For this review, take the finished solid that the model builds, in its own axes (mm). Face numbers are marked on the shaded views. A direction names the side the tool comes from. Coordinates: 2 decimals unless noted, no trailing zeros. Loops run counter-clockwise (first coordinate to the right, second up) from the corner with the lowest first, then second, coordinate; pieces in that order, holes last. Notation, with made-up numbers: (-36, 45.5) -> (-24, 45.5) arc R35 cw to (-24, 84.5) -> close; hole circle Ø4 at (-21.75, 43.25). An arc over 180 degrees is marked (long way). One line per item, written item: value.
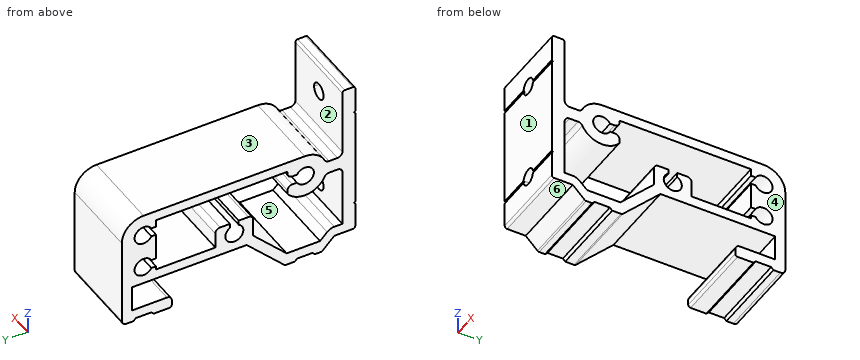
from build123d import *

# Parameters (mm, degrees)
F1_DEPTH = 25.4
F3_DEPTH = 25.4


# Not quite as in the source:
# - ends of sketch curves that miss each other by under 0.0002 mm in the source are joined


with BuildPart() as f1:
    # F0 (on Right) → F1 (new body)
    with BuildSketch(Plane.YZ):
        with BuildLine():
            Line((-36.7665, 26.0985), (-36.7665, 18.2245))
            Line((-36.7665, 18.2245), (-36.3855, 17.8435))
            Line((-36.3855, 17.8435), (-36.7665, 17.4625))
            Line((-36.7665, 17.4625), (-36.7665, -13.5255))
            Line((-36.7665, -13.5255), (-36.3855, -13.9065))
            Line((-36.3855, -13.9065), (-36.7665, -14.2875))
            Line((-36.7665, -14.2875), (-36.7665, -22.1615))
            ThreePointArc((-36.7665, -22.1615), (-36.5433153673, -22.7003153673), (-36.0045, -22.9235))
            Line((-36.0045, -22.9235), (-30.1625, -22.9235))
            Line((-30.1625, -22.9235), (-26.4486898, -26.6373356))
            ThreePointArc((-26.4486898, -26.6373356), (-26.2014589755, -26.8024962038), (-25.9098542, -26.8605))
            Line((-25.9098542, -26.8605), (-24.0665, -26.8605))
            Line((-24.0665, -26.8605), (-23.3045, -26.0985))
            Line((-23.3045, -26.0985), (-18.4785, -26.0985))
            Line((-18.4785, -26.0985), (-17.7165, -26.8605))
            Line((-17.7165, -26.8605), (-14.9389846, -26.8605))
            ThreePointArc((-14.9389846, -26.8605), (-14.6473881211, -26.8024996403), (-14.4001819327, -26.6373280669))
            Line((-14.4001819327, -26.6373280669), (-2.5583642, -14.7955))
            Line((-2.5583642, -14.7955), (33.5915, -14.7955))
            Line((33.5915, -14.7955), (33.5915, -22.9235))
            Line((33.5915, -22.9235), (22.5425, -22.9235))
            ThreePointArc((22.5425, -22.9235), (21.4648692655, -23.3698692655), (21.0185, -24.4475))
            Line((21.0185, -24.4475), (21.0185, -26.0985))
            ThreePointArc((21.0185, -26.0985), (21.2416846327, -26.6373153673), (21.7805, -26.8605))
            Line((21.7805, -26.8605), (26.7335, -26.8605))
            Line((26.7335, -26.8605), (27.4955, -26.0985))
            Line((27.4955, -26.0985), (32.3215, -26.0985))
            Line((32.3215, -26.0985), (33.0835, -26.8605))
            Line((33.0835, -26.8605), (35.2425, -26.8605))
            ThreePointArc((35.2425, -26.8605), (36.3201307345, -26.4141307345), (36.7665, -25.3365))
            Line((36.7665, -25.3365), (36.7665, 1.9685))
            ThreePointArc((36.7665, 1.9685), (34.7578383054, 6.8178383054), (29.9085, 8.8265))
            Line((29.9085, 8.8265), (-20.8915, 8.8265))
            ThreePointArc((-20.8915, 8.8265), (-24.5711182212, 7.7557768852), (-27.1017564824, 4.8779464117))
            ThreePointArc((-27.1017564824, 4.8779464117), (-27.6641193484, 4.2384353631), (-28.4818074, 4.0005))
            Line((-28.4818074, 4.0005), (-31.1785, 4.0005))
            ThreePointArc((-31.1785, 4.0005), (-32.2561307345, 4.4468692655), (-32.7025, 5.5245))
            Line((-32.7025, 5.5245), (-32.7025, 26.0985))
            ThreePointArc((-32.7025, 26.0985), (-32.9256846327, 26.6373153673), (-33.4645, 26.8605))
            Line((-33.4645, 26.8605), (-36.0045, 26.8605))
            ThreePointArc((-36.0045, 26.8605), (-36.5433153673, 26.6373153673), (-36.7665, 26.0985))
        make_face()
        with BuildLine():
            Line((-18.4133236, 3.3655), (-16.9545, 3.3655))
            ThreePointArc((-16.9545, 3.3655), (-15.8768692655, 3.8118692655), (-15.4305, 4.8895))
            Line((-15.4305, 4.8895), (-15.4305, 5.6515))
            Line((-15.4305, 5.6515), (25.9715, 5.6515))
            Line((25.9715, 5.6515), (25.9715, 3.3655))
            Line((25.9715, 3.3655), (27.430349, 3.3655))
            ThreePointArc((27.430349, 3.3655), (32.7533, 1.9685), (27.4303420089, 0.5714960589))
            Line((27.4303420089, 0.5714960589), (25.9715, 0.5715))
            Line((25.9715, 0.5715), (25.9715, -7.747))
            Line((25.9715, -7.747), (27.430349, -7.747))
            ThreePointArc((27.430349, -7.747), (32.7533, -9.144), (27.4303420089, -10.5410039411))
            Line((27.4303420089, -10.5410039411), (25.9715, -10.541))
            Line((25.9715, -10.541), (25.9715, -11.6205))
            Line((25.9715, -11.6205), (7.3025, -11.6205))
            Line((7.3025, -11.6205), (7.3025, -6.731))
            ThreePointArc((7.3025, -6.731), (6.8561307345, -5.6533692655), (5.7785, -5.207))
            Line((5.7785, -5.207), (2.7305, -5.207))
            Line((2.7305, -5.207), (2.7305, -6.665849))
            ThreePointArc((2.7305, -6.665849), (1.3335, -11.9888), (-0.0635039411, -6.6658420089))
            Line((-0.0635039411, -6.6658420089), (-0.0635, -5.207))
            Line((-0.0635, -5.207), (-3.1115, -5.207))
            ThreePointArc((-3.1115, -5.207), (-4.1891307345, -5.6533692655), (-4.6355, -6.731))
            Line((-4.6355, -6.731), (-4.6355, -12.3825))
            Line((-4.6355, -12.3825), (-15.1765, -22.9235))
            Line((-15.1765, -22.9235), (-25.6723642, -22.9235))
            Line((-25.6723642, -22.9235), (-27.9174194, -20.6784448))
            ThreePointArc((-27.9174194, -20.6784448), (-28.9474718056, -19.9901859209), (-30.1625, -19.7485))
            Line((-30.1625, -19.7485), (-32.7025, -19.7485))
            Line((-32.7025, -19.7485), (-32.7025, -1.5875))
            ThreePointArc((-32.7025, -1.5875), (-32.2561307345, -0.5098692655), (-31.1785, -0.0635))
            Line((-31.1785, -0.0635), (-28.4818074, -0.0635))
            ThreePointArc((-28.4818074, -0.0635), (-27.6641096434, -0.3014415336), (-27.1017455591, -0.9409666943))
            ThreePointArc((-27.1017455591, -0.9409666943), (-21.615457962, -4.8511809947), (-15.4305020835, -2.1799534173))
            Line((-15.4305020835, -2.1799534173), (-15.4305, -0.9525))
            ThreePointArc((-15.4305, -0.9525), (-15.8768692655, 0.1251307345), (-16.9545, 0.5715))
            Line((-16.9545, 0.5715), (-18.4133236, 0.5715))
            ThreePointArc((-18.4133236, 0.5715), (-23.7363, 1.9685), (-18.4133236, 3.3655))
        make_face(mode=Mode.SUBTRACT)
    extrude(amount=F1_DEPTH)

    # F2 (on face) → F3 (cut)
    with BuildSketch(Plane.XZ.offset(36.7665)):
        with BuildLine():
            ThreePointArc((10.1889011104, 17.4625), (12.8915839509, 15.311811972), (15.24, 17.8445763886))
            ThreePointArc((15.24, 17.8445763886), (12.5084160491, 20.3773408052), (10.1889011104, 17.4625))
        make_face()
        with BuildLine():
            ThreePointArc((10.1887375685, -13.5255), (12.5089588736, -16.4393054185), (15.24, -13.9065))
            ThreePointArc((15.24, -13.9065), (12.8910411264, -11.3736945815), (10.1887375685, -13.5255))
        make_face()
    extrude(amount=-F3_DEPTH, mode=Mode.SUBTRACT)


solid = f1.part
1. Take a section at B-B, the plane z = 16.5. Give the boundary of the cut face in (x, y).
Return value:
outline: (0, -36.77) -> (10.55, -36.77) -> (10.55, -32.7) -> (0, -32.7) -> close; (14.85, -36.77) -> (25.4, -36.77) -> (25.4, -32.7) -> (14.85, -32.7) -> close
2. Insertion check: pin 1 Ø3 at (x, y) = (5, 6) entering from +Z; pin 2 Ø0.8 at (x, z) = (11, -25.5) entering from -Y; pin 3 Ø5 at (x, y) = (12.5, 18) entering from -Z. Each pin has a flat end and moves straight along its axis. Give the tip position at first contact, or say it passes through.
Return value:
pin 1: stops at z = 8.83
pin 2: stops at y = -27.99
pin 3: stops at z = -14.8
3. Take a section at A-A, the plane z = -9. Give the boundary of the cut face in (x, y).
Return value:
outline: (0, -36.77) -> (25.4, -36.77) -> (25.4, -32.7) -> (0, -32.7) -> close; (0, -4.64) -> (25.4, -4.64) -> (25.4, -1.51) -> (0, -1.51) -> close; (0, 4.17) -> (25.4, 4.17) -> (25.4, 7.3) -> (0, 7.3) -> close; (0, 32.75) -> (25.4, 32.75) -> (25.4, 36.77) -> (0, 36.77) -> close
4. For the marked faces 4, 5 and 6, list the 3-axis set-ups (+Z, -Z, +X, -X, +Y, -Y) from which the entire face can be reached by the end or side of a thin tool; tool diameter is ignored.
Return value:
face 4: +Z, -Z, +X, +Y, -Y
face 5: +X, -X
face 6: -Z, +X, -X, -Y
5. To check wall thickness, follow probe 1 along Y at (x, z) = (1.25, -17.5); probe 2 along Y at (x, z) = (3.75, 0); probe 3 along Z at (x, y) = (24, 1.5). State the ranges of each line that lie inside material, in increasing order. Write a range as from..to.
Return value:
probe 1: y = -36.77..-32.7, -9.75..-5.26, 33.59..36.77
probe 2: y = -36.77..-22.95, -18.84..-15.76, 25.97..27.85, 31.96..36.77
probe 3: z = -14.8..-11.98, 5.65..8.83
6. The part is to be moulded in two halves that separate along Y. For the marked faces 1, 2 and 3, say which applies: pulls with the +Y half, pulls with the -Y half, needs draft (parallel to the pull), parting line crosses it, or undercut.
Return value:
face 1: pulls with the -Y half
face 2: undercut
face 3: needs draft
